```python
from build123d import *

# Parameters (mm, degrees)
F1_DEPTH = 50.8
F3_DEPTH = 101.6


with BuildPart() as f1:
    # F0 (on Right) → F1 (new body)
    with BuildSketch(Plane.YZ):
        with BuildLine():
            ThreePointArc((12.43875, -2.562713), (12.634519, -1.287998), (12.7, 0))
            ThreePointArc((12.7, 0), (12.634519, 1.287998), (12.43875, 2.562713))
            ThreePointArc((12.43875, 2.562713), (10.998523, 6.35), (8.43875, 9.490917))
            ThreePointArc((8.43875, 9.490917), (6.35, 10.998523), (4, 12.05363))
            ThreePointArc((4, 12.05363), (0, 12.7), (-4, 12.05363))
            ThreePointArc((-4, 12.05363), (-6.35, 10.998523), (-8.43875, 9.490917))
            ThreePointArc((-8.43875, 9.490917), (-10.998523, 6.35), (-12.43875, 2.562713))
            ThreePointArc((-12.43875, 2.562713), (-12.7, 0), (-12.43875, -2.562713))
            ThreePointArc((-12.43875, -2.562713), (-10.998523, -6.35), (-8.43875, -9.490917))
            ThreePointArc((-8.43875, -9.490917), (-6.35, -10.998523), (-4, -12.05363))
            ThreePointArc((-4, -12.05363), (0, -12.7), (4, -12.05363))
            ThreePointArc((4, -12.05363), (6.35, -10.998523), (8.43875, -9.490917))
            ThreePointArc((8.43875, -9.490917), (10.998523, -6.35), (12.43875, -2.562713))
        make_face()
        with BuildLine():
            ThreePointArc((8.43875, 9.490917), (10.998523, 6.35), (12.43875, 2.562713))
            Line((12.43875, 2.562713), (15.462624, 6.617949))
            Line((15.462624, 6.617949), (14.462624, 8.35))
            Line((14.462624, 8.35), (13.462624, 10.082051))
            Line((13.462624, 10.082051), (8.43875, 9.490917))
        make_face()
        with BuildLine():
            Line((15.462624, -6.617949), (12.43875, -2.562713))
            ThreePointArc((12.43875, -2.562713), (10.998523, -6.35), (8.43875, -9.490917))
            Line((8.43875, -9.490917), (13.462624, -10.082051))
            Line((13.462624, -10.082051), (14.462624, -8.35))
            Line((14.462624, -8.35), (15.462624, -6.617949))
        make_face()
        with BuildLine():
            ThreePointArc((-4, 12.05363), (0, 12.7), (4, 12.05363))
            Line((4, 12.05363), (2, 16.7))
            Line((2, 16.7), (0, 16.7))
            Line((0, 16.7), (-2, 16.7))
            Line((-2, 16.7), (-4, 12.05363))
        make_face()
        with BuildLine():
            Line((2, -16.7), (4, -12.05363))
            ThreePointArc((4, -12.05363), (0, -12.7), (-4, -12.05363))
            Line((-4, -12.05363), (-2, -16.7))
            Line((-2, -16.7), (0, -16.7))
            Line((0, -16.7), (2, -16.7))
        make_face()
        with BuildLine():
            ThreePointArc((-12.43875, 2.562713), (-10.998523, 6.35), (-8.43875, 9.490917))
            Line((-8.43875, 9.490917), (-13.462624, 10.082051))
            Line((-13.462624, 10.082051), (-14.462624, 8.35))
            Line((-14.462624, 8.35), (-15.462624, 6.617949))
            Line((-15.462624, 6.617949), (-12.43875, 2.562713))
        make_face()
        with BuildLine():
            Line((-13.462624, -10.082051), (-8.43875, -9.490917))
            ThreePointArc((-8.43875, -9.490917), (-10.998523, -6.35), (-12.43875, -2.562713))
            Line((-12.43875, -2.562713), (-15.462624, -6.617949))
            Line((-15.462624, -6.617949), (-14.462624, -8.35))
            Line((-14.462624, -8.35), (-13.462624, -10.082051))
        make_face()
    extrude(amount=F1_DEPTH)

    # F2 (on face) → F3 (cut)
    with BuildSketch(Plane.YZ.offset(50.8)):
        with BuildLine():
            Line((2.077989, 2.300426), (-2.077989, 2.300426))
            ThreePointArc((-2.077989, 2.300426), (0, -3.1), (2.077989, 2.300426))
        make_face()
    extrude(amount=-F3_DEPTH, mode=Mode.SUBTRACT)


solid = f1.part
```
Design review of the part built by this model. Coordinates are the model's own, in mm. A direction names the side the tool comes from. Round coordinates to 2 decimals unless told otherwise and drop trailing zeros. Write each loop counter-clockwise with the first axis right and the second up, starting at its lowest first coordinate (ties: lowest second). Pieces come first, ordered by that corner, then holes. Notation, with made-up numbers: (5.25, -18) -> (30.25, -18) arc R34 ccw to (30.25, 20) -> close; hole circle Ø8 at (15.25, 62.5). An arc over 180 degrees is marked (long way). Write item = value, one per line. Start each with the question number.
1) Clearance check with flat-ended pins moving along their axes: pin 1 (10 mm diameter, centred on x = 12.5, z = -13, fed in from -Y); pin 2 (3 mm diameter, centred on x = 24, y = 8.5, fed in from -Z); pin 3 (10 mm diameter, centred on x = 39.5, z = -0.5, fed in from -Y). State where each tip first meets the part, or that it passes through.
2) Take a section at A-A, the plane x = 45. State the section outline as (y, z) points.
3) Take a section at C-C, the plane z = 6. State the section outline as (x, y) points, plus the area to 3 significant figures.
4) Tool access review of faces 1 (the face through (26, 0, 2.3)), 2 (the face through (25.04, -13.93, -4.56)), 3 (the face through (25.044, -6.319, 11.017)), 4 (the face through (25.044, 10.916, -9.782)): name each direction out of +Z, -Z, +X, -X, +Y, -Y from which nothing blocks a thin tool from reaching the whole face with its end or side.
5) Wall thickness on probe 1 along Z at (x, y) = (18.5, 0); probe 2 along Z at (x, y) = (39, 13.5); probe 3 along Z at (x, y) = (14, 6): over which ranges is each line inside the solid? List them lowest first. Write a range as from..to.
6) Mouldability with a two-part tool opening along Z and no side actions: class faces 5 (the face through (25.04, -14.45, 8.37)), 6 (the face through (25, 0, -16.7)), 7 (the face through (25.044, 13.972, -4.619)) as +Z half, -Z half, draft (parallel to the pull), parting line (faces both ways), or undercut.
7) Take a section at D-D, the plane y = 7.5. State the section outline as (x, z) points, plus the area to 3 significant figures.
8) Take a section at B-B, the plane y = 0. State the section outline as (x, z) points, plus the area to 3 significant figures.
Results list:
q1.pin_1 = -14.66
q1.pin_2 = -10.6
q1.pin_3 = -14.63
q2.outline = (-15.46, -6.62) -> (-13.46, -10.08) -> (-8.44, -9.49) arc R12.7 ccw to (-4, -12.05) -> (-2, -16.7) -> (2, -16.7) -> (4, -12.05) arc R12.7 ccw to (8.44, -9.49) -> (13.46, -10.08) -> (15.46, -6.62) -> (12.44, -2.56) arc R12.7 ccw to (12.7, 0) arc R12.7 ccw to (12.44, 2.56) -> (15.46, 6.62) -> (13.46, 10.08) -> (8.44, 9.49) arc R12.7 ccw to (4, 12.05) -> (2, 16.7) -> (-2, 16.7) -> (-4, 12.05) arc R12.7 ccw to (-8.44, 9.49) -> (-13.46, 10.08) -> (-15.46, 6.62) -> (-12.44, 2.56) arc R12.7 ccw to (-12.44, -2.56) -> close; hole (-2.08, 2.3) arc R3.1 ccw (long way) to (2.08, 2.3) -> close
q3.outline = (0, -15) -> (50.8, -15) -> (50.8, 15) -> (0, 15) -> close
q3.area = 1,520 mm²
q4.face_1 = +X, -X
q4.face_2 = +X, -X, -Y
q4.face_3 = +Z, +X, -X
q4.face_4 = -Z, +X, -X
q5.probe_1 = -16.7..-3.1, 2.3..16.7
q5.probe_2 = -10.02..-3.99, 3.99..10.02
q5.probe_3 = -11.19..11.19
q6.face_5 = +Z half
q6.face_6 = -Z half
q6.face_7 = undercut
q7.outline = (0, -10.25) -> (50.8, -10.25) -> (50.8, 10.25) -> (0, 10.25) -> close
q7.area = 1,040 mm²
q8.outline = (0, -16.7) -> (50.8, -16.7) -> (50.8, -3.1) -> (0, -3.1) -> close; (0, 2.3) -> (50.8, 2.3) -> (50.8, 16.7) -> (0, 16.7) -> close
q8.area = 1,420 mm²
